Part model, mm, in its own coordinate system. Face numbers are marked on the shaded views. A direction names the side the tool comes from. Give positions to 0.01 mm unless a question says otherwise; leave off trailing zeros. Write each loop counter-clockwise with the first axis right and the second up, starting at its lowest first coordinate (ties: lowest second). Pieces come first, ordered by that corner, then holes. Notation, with made-up numbers: (31, 24) - (83, 24) arc R25 cw to (83, 56) - close; hole circle Ø10 at (39, -35.75). An arc over 180 degrees is marked (long way). Answer in a Markdown table with one row per item. Add a question column.
1. Pull direction Y, two halves, no side cores. Call the marked faces 4, 5, 6 and 7: released by +Y, released by -Y, zero draft, split by the parting line, or undercut.
2. Drop flat-ended pins along their axis: pin 1 Ø1.6 at (x, z) = (26.5, 2) entering from -Y; pin 2 Ø3.5 at (y, z) = (-3.5, 2) entering from -X; pin 3 Ø3 at (y, z) = (5.5, 4.5) entering from -X. Give the stop position or say it passes through.
3. Probe line 1 along Y through (x, z) = (3.5, 6.25); line 2 along X through (y, z) = (56, 5.5); line 3 along Y through (x, z) = (32.2, 2.75). List the from-to ranges inside material, lowest first.
4. Band-saw the part on D-D on z = 4.25. State how many separate pieces and enclosed holes the cut face has, plus the area to 3 significant figures.
5. Band-saw the part on C-C on y = 50.5. Write the cut outline in (x, z), plus the area to 3 significant figures.
6. Band-saw the part on B-B on x = 58.2. Write the cut outline in (y, z).
7. Band-saw the part on A-A on y = 61. Write the cut outline in (x, z), plus the area to 3 significant figures.
8. Which spindle directions (+Z, -Z, +X, -X, +Y, -Y) get a long thin tool onto all of the face, cutting with end or side? Do the marked faces 1, 2 and 3. Say none if no direction does.
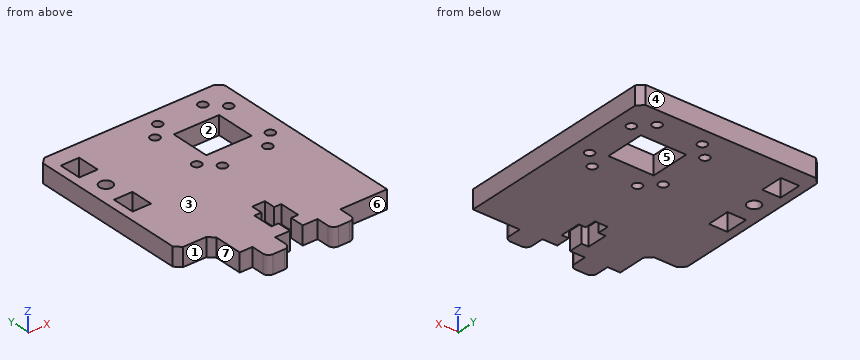
Autodesk Inventor part; units mm, degrees
ref_plane "YZ Plane" through (0, 0, 0) normal (1, 0, 0) x (0, 1, 0)
ref_plane "XZ Plane" through (0, 0, 0) normal (0, 1, 0) x (-1, 0, 0)
ref_plane "XY Plane" through (0, 0, 0) normal (0, 0, 1) x (1, 0, 0)
sketch "Sketch1" plane through (0, 0, 0) normal (0, 0, 1) x (1, 0, 0)
  line L0 (12.2, 0) -> (64.2, 0)
  line L1 (64.2, 0) -> (64.2, 72)
  line L2 (64.2, 72) -> (0, 72)
  line L3 (0, 72) -> (0, 12)
  line L4 (3, 66) -> (9.5, 66)
  line L5 (9.5, 66) -> (9.5, 58)
  line L6 (9.5, 58) -> (3, 58)
  line L7 (3, 58) -> (3, 66)
  line L8 (3, 43) -> (9.5, 43)
  line L9 (9.5, 43) -> (9.5, 35)
  line L10 (9.5, 35) -> (3, 35)
  line L11 (3, 35) -> (3, 43)
  line L12 (0, 12) -> (12.2, 12)
  line L13 (12.2, 12) -> (12.2, 0)
  line L14 (3, 58) -> (9.5, 43) construction
  line L15 (3, 43) -> (9.5, 58) construction
  circle A0 centre (6.25, 50.5) radius 2.25
  point P0 (0, 0)
  dimension "d1" = 6.5
  dimension "d2" = 8
  dimension "d3" = 8
  dimension "d4" = 15
  dimension "d5" = 3
  dimension "d6" = 72
  dimension "d7" = 4.5
  dimension "d8" = 64.2
  dimension "d9" = 12
  dimension "d10" = 52
  dimension "d11" = 6
extrude "Extrusion1" add sketch "Sketch1" along normal blind 6.5
sketch "Sketch2" plane through (0, 0, 6.5) normal (0, 0, 1) x (1, 0, 0)
  line L0 (64.2, 0) -> (64.2, 72)
  line L1 (12.2, 0) -> (64.2, 0)
  line L2 (29.95, 16.3) -> (34.45, 16.3)
  line L3 (34.45, 0) -> (29.95, 0)
  line L4 (36.95, 12.3) -> (36.95, 5)
  line L5 (27.45, 5) -> (27.45, 12.3)
  line L6 (29.95, 0) -> (29.95, 5)
  line L7 (29.95, 12.3) -> (29.95, 16.3)
  line L8 (27.45, 12.3) -> (29.95, 12.3)
  line L9 (34.45, 12.3) -> (36.95, 12.3)
  line L10 (34.45, 16.3) -> (34.45, 12.3)
  line L11 (34.45, 5) -> (34.45, 0)
  line L12 (36.95, 5) -> (34.45, 5)
  line L13 (29.95, 5) -> (27.45, 5)
  point P0 (0, 0)
  point P1 (32.2, 16.3)
  dimension "d14" = 2.5
  dimension "d15" = 2.5
  dimension "d16" = 4.5
  dimension "d17" = 5
  dimension "d18" = 7.3
  dimension "d19" = 4
  dimension "d20" = 32
extrude "Extrusion2" cut sketch "Sketch2" against normal blind 6.5
sketch "Sketch3" plane through (0, 0, 6.5) normal (0, 0, 1) x (1, 0, 0)
  line L0 (34.45, 0) -> (64.2, 0)
  line L1 (12.2, 0) -> (29.95, 0)
  line L2 (29.95, 16.3) -> (34.45, 16.3)
  line L3 (16.7, 0) -> (24.7, 0)
  line L4 (24.7, 0) -> (24.7, -4.5)
  line L5 (22.7, -6.5) -> (18.7, -6.5)
  line L6 (16.7, -4.5) -> (16.7, 0)
  line L7 (39.7, 0) -> (47.7, 0)
  line L8 (47.7, 0) -> (47.7, -4.5)
  line L9 (45.7, -6.5) -> (41.7, -6.5)
  line L10 (39.7, -4.5) -> (39.7, 0)
  arc A0 (16.7, -4.5) -> (18.7, -6.5) centre (18.7, -4.5) ccw
  arc A1 (22.7, -6.5) -> (24.7, -4.5) centre (22.7, -4.5) ccw
  arc A2 (39.7, -4.5) -> (41.7, -6.5) centre (41.7, -4.5) ccw
  arc A3 (45.7, -6.5) -> (47.7, -4.5) centre (45.7, -4.5) ccw
  point P0 (0, 0)
  point P1 (32.2, 16.3)
  dimension "d23" = 2
  dimension "d24" = 8
  dimension "d25" = 8
  dimension "d26" = 6.5
  dimension "d27" = 15
  dimension "d28" = 7.5
extrude "Extrusion3" add sketch "Sketch3" against normal blind 6.5
chamfer "Chamfer1" distance 2 angle 45 2 edges at (0, 72, 3.25) (64.2, 72, 3.25)
sketch "Sketch4" plane through (0, 0, 0) normal (0, 0, -1) x (-1, 0, 0)
  line L0 (-64.2, 70) -> (-64.2, 0)
  line L1 (-2, 72) -> (-62.2, 72)
  line L2 (-37.2, 59) -> (-53.2, 59)
  line L3 (-53.2, 59) -> (-53.2, 45)
  line L4 (-53.2, 45) -> (-37.2, 45)
  line L5 (-37.2, 45) -> (-37.2, 59)
  line L6 (-32.2, 66) -> (-58.2, 66) construction
  line L7 (-58.2, 66) -> (-58.2, 38) construction
  line L8 (-58.2, 38) -> (-32.2, 38) construction
  line L9 (-32.2, 38) -> (-32.2, 66) construction
  circle A0 centre (-58.2, 61) radius 1.6
  circle A1 centre (-58.2, 43) radius 1.6
  circle A2 centre (-53.2, 38) radius 1.6
  circle A3 centre (-37.2, 38) radius 1.6
  circle A4 centre (-32.2, 43) radius 1.6
  circle A5 centre (-32.2, 61) radius 1.6
  circle A6 centre (-37.2, 66) radius 1.6
  circle A7 centre (-53.2, 66) radius 1.6
  point P0 (0, 0)
  point P1 (-58.2, 52)
  point P2 (-53.2, 52)
  point P3 (-45.2, 38)
  point P4 (-45.2, 45)
  dimension "d34" = 3.2
  dimension "d35" = 5
  dimension "d36" = 5
  dimension "d37" = 5
  dimension "d38" = 5
  dimension "d39" = 5
  dimension "d40" = 5
  dimension "d41" = 5
  dimension "d42" = 5
  dimension "d43" = 16
  dimension "d44" = 14
  dimension "d45" = 5
  dimension "d46" = 7
  dimension "d47" = 6
  dimension "d48" = 6
extrude "Extrusion4" cut sketch "Sketch4" against normal through all
chamfer "Chamfer2" distance 2 angle 45 2 edges at (0, 12, 3.25) (12.2, 12, 3.25)
equation "\"d36\" = d35"
equation "\"d37\" = d35"
equation "\"d38\" = d35"
equation "\"d39\" = d35"
equation "\"d40\" = d35"
equation "\"d41\" = d35"
equation "\"d42\" = d35"
properties part number "x_motor_cable_mount" material "Plywood, Finish"
Values:
| question | item | result |
|---|---|---|
| 1 | face 4 | released by +Y |
| 1 | face 5 | undercut |
| 1 | face 6 | released by -Y |
| 1 | face 7 | zero draft |
| 2 | pin 1 | stops at y = 0 |
| 2 | pin 2 | stops at x = 16.7 |
| 2 | pin 3 | stops at x = 12.2 |
| 3 | line 1 | y = 12 to 35, 43 to 58, 66 to 72 |
| 3 | line 2 | x = 0 to 37.2, 53.2 to 64.2 |
| 3 | line 3 | y = 16.3 to 41.4, 44.6 to 59.4, 62.6 to 72 |
| 4 | separate pieces | 1 |
| 4 | enclosed holes | 12 |
| 4 | area | 4,050 mm² |
| 5 | outline | (0, 0) - (4, 0) - (4, 6.5) - (0, 6.5) - close; (8.5, 0) - (37.2, 0) - (37.2, 6.5) - (8.5, 6.5) - close; (53.2, 0) - (64.2, 0) - (64.2, 6.5) - (53.2, 6.5) - close |
| 5 | area | 284 mm² |
| 6 | outline | (0, 0) - (41.4, 0) - (41.4, 6.5) - (0, 6.5) - close; (44.6, 0) - (59.4, 0) - (59.4, 6.5) - (44.6, 6.5) - close; (62.6, 0) - (72, 0) - (72, 6.5) - (62.6, 6.5) - close |
| 7 | outline | (0, 0) - (3, 0) - (3, 6.5) - (0, 6.5) - close; (9.5, 0) - (30.6, 0) - (30.6, 6.5) - (9.5, 6.5) - close; (33.8, 0) - (56.6, 0) - (56.6, 6.5) - (33.8, 6.5) - close; (59.8, 0) - (64.2, 0) - (64.2, 6.5) - (59.8, 6.5) - close |
| 7 | area | 333 mm² |
| 8 | face 1 | +Z, -Z, -X, -Y |
| 8 | face 2 | +Z, -Z |
| 8 | face 3 | +Z, +X, -X, +Y, -Y |
